Autodesk Inventor part; units mm, degrees
ref_plane "YZ Plane" through (0, 0, 0) normal (1, 0, 0) x (0, 1, 0)
ref_plane "XZ Plane" through (0, 0, 0) normal (0, 1, 0) x (-1, 0, 0)
ref_plane "XY Plane" through (0, 0, 0) normal (0, 0, 1) x (1, 0, 0)
sketch "Sketch1" plane through (0, 0, 0) normal (0, 0, 1) x (1, 0, 0)
  circle A0 centre (0, 0) radius 25.4
  dimension "d0" = 50.8
extrude "Extrusion1" add sketch "Sketch1" along normal blind 25.4
sketch "Sketch2" plane through (0, 0, 25.4) normal (0, 0, 1) x (1, 0, 0)
  arc A0 (27.94, 31.75) -> (-27.94, 31.75) centre (0, 31.75) ccw
  arc A1 (-46.9331, -19.4403) -> (46.9331, -19.4403) centre (0, 0) ccw
  line L0 (-27.94, 31.75) -> (-27.94, -11.5731)
  line L1 (-27.94, -11.5731) -> (-46.9331, -19.4403)
  line L2 (27.94, 31.75) -> (27.94, -11.5731)
  line L3 (27.94, -11.5731) -> (46.9331, -19.4403)
  circle A2 centre (0, 0) radius 25.4
  dimension "d3" = 31.75
  dimension "d4" = 50.8
  dimension "d5" = 27.94
  dimension "d6" = 135
extrude "Extrusion2" add sketch "Sketch2" along normal blind 6.35 contours L2 L3 A1 L1 L0 A0 | A2
sketch "Sketch3" plane through (0, 0, 31.75) normal (0, 0, 1) x (1, 0, 0)
  circle A0 centre (0, 31.75) radius 25.4
  arc A1 (27.94, 31.75) -> (-27.94, 31.75) centre (0, 31.75) ccw
  point P0 (0, 0)
  dimension "d9" = 50.8
extrude "Extrusion3" add sketch "Sketch3" along normal blind 20.32
pattern_linear "Rectangular Pattern1" count 2 spacing 26.67 along (0, 0, 1) of "Extrusion2"
sketch "Sketch4" plane through (0, 0, 58.42) normal (0, 0, 1) x (1, 0, 0)
  circle A0 centre (0, 0) radius 25.4
  dimension "d15" = 50.8
extrude "Extrusion4" add sketch "Sketch4" along normal blind 50.8
sketch "Sketch5" plane through (0, 4.445, 109.22) normal (0, 0, 1) x (-1, 0, 0)
  arc A0 (27.94, 36.195) -> (-27.94, 36.195) centre (0, 36.195) ccw
  arc A1 (-46.9331, -14.9953) -> (46.9331, -14.9953) centre (0, 4.445) ccw
  line L0 (-27.94, 36.195) -> (-27.94, -7.1281)
  line L1 (-27.94, -7.1281) -> (-46.9331, -14.9953)
  line L2 (27.94, 36.195) -> (27.94, -7.1281)
  line L3 (27.94, -7.1281) -> (46.9331, -14.9953)
  circle A2 centre (0, 4.445) radius 25.4
  point P0 (0, 4.445)
  dimension "d19" = 50.8
  dimension "d20" = 27.94
  dimension "d18" = 135
  dimension "d25" = 31.75
extrude "Extrusion5" add sketch "Sketch5" along normal blind 6.35 contours L2 L3 A1 L1 L0 A0 | A2
sketch "Sketch6" plane through (0, 4.445, 115.57) normal (0, 0, 1) x (1, 0, 0)
  circle A0 centre (0, -36.195) radius 25.4
  arc A1 (-27.94, -36.195) -> (27.94, -36.195) centre (0, -36.195) ccw
  point P0 (0, -4.445)
  dimension "d26" = 50.8
extrude "Extrusion6" add sketch "Sketch6" along normal blind 25.4
pattern_linear "Rectangular Pattern2" count 2 spacing 26.67 along (0, 0, 1) of "Extrusion5"
sketch "Sketch7" plane through (0, 0, 142.24) normal (0, 0, 1) x (1, 0, 0)
  circle A0 centre (0, 0) radius 25.4
  dimension "d32" = 50.8
extrude "Extrusion7" add sketch "Sketch7" along normal blind 25.4
sketch "Sketch8" plane through (0, 0, 167.64) normal (0, 0, 1) x (1, 0, 0)
  circle A0 centre (0, 0) radius 12.7
  dimension "d35" = 25.4
extrude "Extrusion8" add sketch "Sketch8" along normal blind 25.4
properties part number "crankshaft"
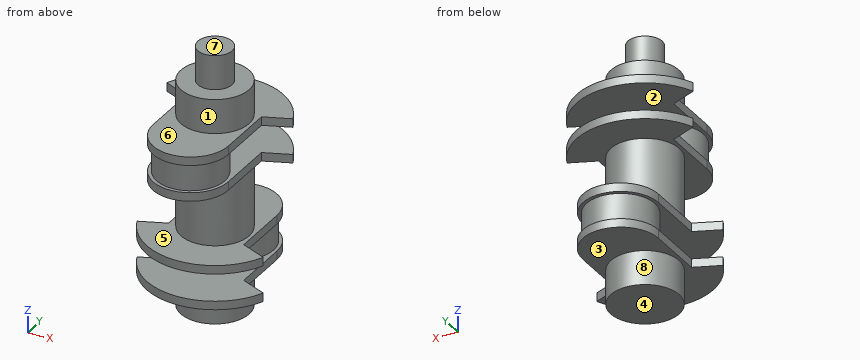
Part model, mm, in its own coordinate system. Face numbers are marked on the shaded views. A direction names the side the tool comes from. Coordinates: 2 decimals unless noted, no trailing zeros. Write each loop counter-clockwise with the first axis right and the second up, starting at its lowest first coordinate (ties: lowest second). Pieces come first, ordered by that corner, then holes.
Item 1: Which spindle directions (+Z, -Z, +X, -X, +Y, -Y) get a long thin tool onto all of the face, cutting with end or side? Do the marked faces 4, 5, 6, 7 and 8. Say none if no direction does.
Item 2: Slice it at D-D (z = 34). Write the cut outline in (x, y).
Item 3: Mould opens along Z. For the marked faces 1, 2 and 3 say: released by +Z, released by -Z, zero draft, split by the parting line, or undercut.
Item 4: Slice it at C-C (x = 40.5). Write the cut outline in (y, z), and give its area (3 significant figures).
Item 5: Probe line 1 (Z direction, x = -27, y = 2); line 2 (Z direction, x = 15, y = 24.5); line 3 (Z direction, x = 5, y = 0). List the from-to ranges inside material, lowest first.
Item 6: Pin check, flat tips, straight feed: pin 1 (10 mm diameter, centred on x = -26, z = 134, fed in from +Y); pin 2 (1.9 mm diameter, centred on y = -0.5, z = 56.5, fed in from +X); pin 3 (1 mm diameter, centred on x = 13.5, z = 73, fed in from -Y). Stop position of each tip, or through.
Item 7: Slice it at A-A (y = 44). Write the cut outline in (x, z), and give its area (3 significant figures).
Results found:
1. face 4: -Z, +X, -X, +Y, -Y
1. face 5: none
1. face 6: +Z
1. face 7: +Z, +X, -X, +Y, -Y
1. face 8: -Z
2. outline: circle Ø50.8 at (0, 31.75)
3. face 1: zero draft
3. face 2: undercut
3. face 3: released by -Z
4. outline: (-30.67, 25.4) - (-16.78, 25.4) - (-16.78, 31.75) - (-30.67, 31.75) - close; (-30.67, 52.07) - (-16.78, 52.07) - (-16.78, 58.42) - (-30.67, 58.42) - close; (16.78, 109.22) - (30.67, 109.22) - (30.67, 115.57) - (16.78, 115.57) - close; (16.78, 135.89) - (30.67, 135.89) - (30.67, 142.24) - (16.78, 142.24) - close
4. area: 353 mm2
5. line 1: z = 25.4 to 31.75, 52.07 to 58.42, 109.22 to 115.57, 135.89 to 142.24
5. line 2: z = 25.4 to 58.42, 109.22 to 115.57, 135.89 to 142.24
5. line 3: z = 0 to 31.75, 52.07 to 115.57, 135.89 to 193.04
6. pin 1: stops at y = 46.09
6. pin 2: stops at x = 27.94
6. pin 3: stops at y = -21.82
7. outline: (-25.39, 109.22) - (25.39, 109.22) - (25.39, 115.57) - (-25.39, 115.57) - close; (-25.39, 135.89) - (25.39, 135.89) - (25.39, 142.24) - (-25.39, 142.24) - close; (-25.11, 25.4) - (25.11, 25.4) - (25.11, 31.75) - (22.25, 31.75) - (22.25, 52.07) - (25.11, 52.07) - (25.11, 58.42) - (-25.11, 58.42) - (-25.11, 52.07) - (-22.25, 52.07) - (-22.25, 31.75) - (-25.11, 31.75) - close
7. area: 2,190 mm2
